```python
from build123d import *

# Parameters (mm, degrees)
SKETCH1_W                   = 180
SKETCH1_H                   = 140
BOSS_EXTRUDE1_DEPTH         = 42.5
CUT_EXTRUDE1_DEPTH          = 36
FILLET1_R                   = 2
FILLET2_R                   = 13
FILLET3_R                   = 10
BOSS_EXTRUDE2_DEPTH         = 2
F_6_5_6_5_DIAMETER_HOLE1_D  = 6.5
M5_TAPPED_HOLE1_D           = 4.2
M5_TAPPED_HOLE1_DEPTH       = 14
M5_TAPPED_HOLE1_CBORE_D     = 5
M5_TAPPED_HOLE1_CBORE_DEPTH = 10
M5_TAPPED_HOLE1_TIP         = 1.2618073
BOSS_EXTRUDE3_DEPTH         = 5
SKETCH18_R                  = 6
CUT_EXTRUDE4_DEPTH          = 32.5


with BuildPart() as part:
    # Sketch1 → Boss-Extrude1 (new body)
    with BuildSketch(Plane.XY):
        Rectangle(SKETCH1_W, SKETCH1_H)
    extrude(amount=BOSS_EXTRUDE1_DEPTH)

    # Sketch2 → Cut-Extrude1 (cut)
    with BuildSketch(Plane.XY.offset(42.5)):
        Polygon((-69, 65), (69, 65), (69, 34), (85.5, 34), (85.5, -34), (69, -34), (69, -65), (-69, -65), (-69, -34), (-85.5, -34), (-85.5, 34), (-69, 34), align=None)
    extrude(amount=-CUT_EXTRUDE1_DEPTH, mode=Mode.SUBTRACT)

    # Fillet1
    fillet1_edges = [part.edges().sort_by_distance(p)[0] for p in [
        (-69, 65, 24.5),
        (69, 65, 24.5),
        (85.5, 34, 24.5),
        (85.5, -34, 24.5),
        (69, -65, 24.5),
        (-69, -65, 24.5),
        (-85.5, -34, 24.5),
        (-85.5, 34, 24.5),
    ]]
    fillet(fillet1_edges, radius=FILLET1_R)

    # Fillet2
    fillet2_edges = [part.edges().sort_by_distance(p)[0] for p in [
        (-69, 34, 24.5),
        (69, 34, 24.5),
        (69, -34, 24.5),
        (-69, -34, 24.5),
    ]]
    fillet(fillet2_edges, radius=FILLET2_R)

    # Fillet3
    fillet3_edges = [part.edges().sort_by_distance(p)[0] for p in [
        (-90, 70, 21.25),
        (90, 70, 21.25),
        (90, -70, 21.25),
        (-90, -70, 21.25),
    ]]
    fillet(fillet3_edges, radius=FILLET3_R)

    # Sketch3 → Boss-Extrude2 (add)
    with BuildSketch(Plane.XY.offset(42.5)):
        with BuildLine():
            Line((-71, 63), (-71, 47))
            ThreePointArc((-71, 47), (-74.221825407, 39.221825407), (-82, 36))
            Line((-82, 36), (-83.5, 36))
            ThreePointArc((-83.5, 36), (-86.328427125, 34.828427125), (-87.5, 32))
            Line((-87.5, 32), (-87.5, -32))
            ThreePointArc((-87.5, -32), (-86.328427125, -34.828427125), (-83.5, -36))
            Line((-83.5, -36), (-82, -36))
            ThreePointArc((-82, -36), (-74.221825407, -39.221825407), (-71, -47))
            Line((-71, -47), (-71, -63))
            ThreePointArc((-71, -63), (-69.828427125, -65.828427125), (-67, -67))
            Line((-67, -67), (67, -67))
            ThreePointArc((67, -67), (69.828427125, -65.828427125), (71, -63))
            Line((71, -63), (71, -47))
            ThreePointArc((71, -47), (74.221825407, -39.221825407), (82, -36))
            Line((82, -36), (83.5, -36))
            ThreePointArc((83.5, -36), (86.328427125, -34.828427125), (87.5, -32))
            Line((87.5, -32), (87.5, 32))
            ThreePointArc((87.5, 32), (86.328427125, 34.828427125), (83.5, 36))
            Line((83.5, 36), (82, 36))
            ThreePointArc((82, 36), (74.221825407, 39.221825407), (71, 47))
            Line((71, 47), (71, 63))
            ThreePointArc((71, 63), (69.828427125, 65.828427125), (67, 67))
            Line((67, 67), (-67, 67))
            ThreePointArc((-67, 67), (-69.828427125, 65.828427125), (-71, 63))
        make_face()
        with BuildLine():
            Line((-83.5, -34), (-82, -34))
            ThreePointArc((-82, -34), (-72.807611845, -37.807611845), (-69, -47))
            Line((-69, -47), (-69, -63))
            ThreePointArc((-69, -63), (-68.414213562, -64.414213562), (-67, -65))
            Line((-67, -65), (67, -65))
            ThreePointArc((67, -65), (68.414213562, -64.414213562), (69, -63))
            Line((69, -63), (69, -47))
            ThreePointArc((69, -47), (72.807611845, -37.807611845), (82, -34))
            Line((82, -34), (83.5, -34))
            ThreePointArc((83.5, -34), (84.914213562, -33.414213562), (85.5, -32))
            Line((85.5, -32), (85.5, 32))
            ThreePointArc((85.5, 32), (84.914213562, 33.414213562), (83.5, 34))
            Line((83.5, 34), (82, 34))
            ThreePointArc((82, 34), (72.807611845, 37.807611845), (69, 47))
            Line((69, 47), (69, 63))
            ThreePointArc((69, 63), (68.414213562, 64.414213562), (67, 65))
            Line((67, 65), (-67, 65))
            ThreePointArc((-67, 65), (-68.414213562, 64.414213562), (-69, 63))
            Line((-69, 63), (-69, 47))
            ThreePointArc((-69, 47), (-72.807611845, 37.807611845), (-82, 34))
            Line((-82, 34), (-83.5, 34))
            ThreePointArc((-83.5, 34), (-84.914213562, 33.414213562), (-85.5, 32))
            Line((-85.5, 32), (-85.5, -32))
            ThreePointArc((-85.5, -32), (-84.914213562, -33.414213562), (-83.5, -34))
        make_face(mode=Mode.SUBTRACT)
    extrude(amount=BOSS_EXTRUDE2_DEPTH)

    # Ø6.5 (6.5) Diameter Hole1 (through all)
    with Locations(Plane.XY.offset(42.5)):
        with Locations((-80, 45), (-80, -45), (80, -45), (80, 45)):
            Hole(F_6_5_6_5_DIAMETER_HOLE1_D / 2)

    # M5 Tapped Hole1
    with Locations(Plane.XY.offset(42.5)):
        with Locations((-80, 60), (-80, -60), (80, -60), (80, 60)):
            CounterBoreHole(M5_TAPPED_HOLE1_D / 2, M5_TAPPED_HOLE1_CBORE_D / 2, M5_TAPPED_HOLE1_CBORE_DEPTH, depth=M5_TAPPED_HOLE1_DEPTH)
            with Locations((0, 0, -(M5_TAPPED_HOLE1_DEPTH + M5_TAPPED_HOLE1_TIP / 2))):  # 118° drill point
                Cone(0, M5_TAPPED_HOLE1_D / 2, M5_TAPPED_HOLE1_TIP, mode=Mode.SUBTRACT)

    # Sketch13 → Boss-Extrude3 (add)
    with BuildSketch(Plane.XY.offset(6.5)):
        with BuildLine():
            Line((-69, 47), (-69, -47))
            ThreePointArc((-69, -47), (-72.807611845, -37.807611845), (-82, -34))
            Line((-82, -34), (-83.5, -34))
            ThreePointArc((-83.5, -34), (-84.914213562, -33.414213562), (-85.5, -32))
            Line((-85.5, -32), (-85.5, 32))
            ThreePointArc((-85.5, 32), (-84.914213562, 33.414213562), (-83.5, 34))
            Line((-83.5, 34), (-82, 34))
            ThreePointArc((-82, 34), (-72.807611845, 37.807611845), (-69, 47))
        make_face()
        with BuildLine():
            Line((69, 47), (69, -47))
            ThreePointArc((69, -47), (72.807611845, -37.807611845), (82, -34))
            Line((82, -34), (83.5, -34))
            ThreePointArc((83.5, -34), (84.914213562, -33.414213562), (85.5, -32))
            Line((85.5, -32), (85.5, 32))
            ThreePointArc((85.5, 32), (84.914213562, 33.414213562), (83.5, 34))
            Line((83.5, 34), (82, 34))
            ThreePointArc((82, 34), (72.807611845, 37.807611845), (69, 47))
        make_face()
    extrude(amount=BOSS_EXTRUDE3_DEPTH)

    # Sketch18 → Cut-Extrude4 (cut)
    with BuildSketch(Plane.XY.offset(42.5)):
        with Locations((-80, 45)):
            Circle(SKETCH18_R)
        with Locations((-80, -45)):
            Circle(SKETCH18_R)
        with Locations((80, -45)):
            Circle(SKETCH18_R)
        with Locations((80, 45)):
            Circle(SKETCH18_R)
    extrude(amount=-CUT_EXTRUDE4_DEPTH, mode=Mode.SUBTRACT)


solid = part.part
```
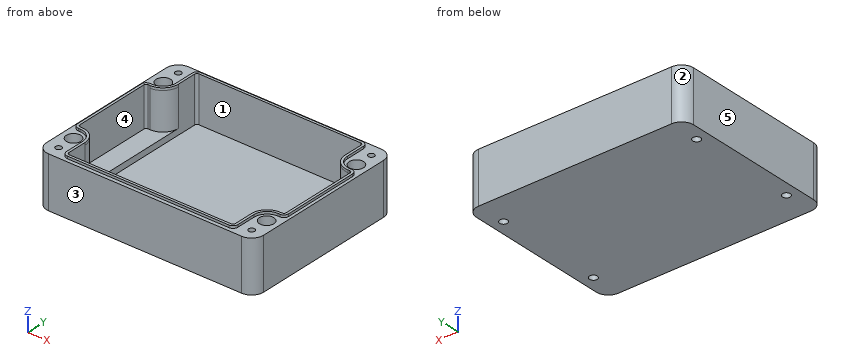
Read the model definition and answer for the solid it produces. Units are mm, in the model's axes. Face numbers are marked on the shaded views. A direction names the side the tool comes from. Give positions to 0.01 mm unless a question says otherwise; leave off trailing zeros. Order: outer loops, then holes, each group sorted by start corner. A loop starts at its lowest first (then second) coordinate and runs counter-clockwise, first axis right, second up.
(1) For the marked faces 1 and 2, determine the directions among +Z, -Z, +X, -X, +Y, -Y from which every point of the face is accessible in a straight line to the end or side of a thin tool.
(2) Given pin 1 (12 mm diameter, centred on x = -31, y = 37.5, fed in from -Z); pin 2 (1.2 mm diameter, centred on x = 83, z = 43.5, fed in from +Y); pin 3 (8 mm diameter, centred on x = 76, y = 0.5, fed in from +Z); pin 4 (3.5 mm diameter, centred on x = -82.5, y = -46.5, fed in from +Z), each flat-ended and moving along its own axis, determine where each tip first touches the part or whether it passes through.
(3) For a pull along X with two mould halves and no side action, classify the marked faces 3, 4 and 5 as released by +X, released by -X, zero draft, split by the parting line, or undercut.
(4) Straight lines are drawn through the part: L1, parallel to Y at x = 80, z = 5; L2, parallel to X at y = 60, z = 31.45; L3, parallel to X at y = -57, z = 42. For each, find the intervals that lie inside material, in ascending order.
(5) Find section B-B (y = -45). Give the number of separate pieces and of enclosed holes in the cut face, plus the area to 3 significant figures.
(6) Find section A-A (x = -27). Give the vertices of the cut face in (y, z), plus the area to 3 significant figures.
Result sheet:
1. face 1: +Z
1. face 2: +Z, -Z, -X, +Y
2. pin 1: stops at z = 0
2. pin 2: stops at y = 36
2. pin 3: stops at z = 11.5
2. pin 4: stops at z = 10
3. face 3: zero draft
3. face 4: undercut
3. face 5: released by -X
4. L1: y = -70 to -48.25, -41.75 to 41.75, 48.25 to 70
4. L2: x = -90 to -82.1, -77.9 to -69, 69 to 77.9, 82.1 to 90
4. L3: x = -90 to -69, 69 to 90
5. separate pieces: 3
5. enclosed holes: 0
5. area: 1,770 mm2
6. outline: (-70, 0) - (70, 0) - (70, 42.5) - (67, 42.5) - (67, 44.5) - (65, 44.5) - (65, 6.5) - (-65, 6.5) - (-65, 44.5) - (-67, 44.5) - (-67, 42.5) - (-70, 42.5) - close
6. area: 1,280 mm2
